The model under review builds one solid part; all positions refer to its coordinate system, in mm. Face numbers are marked on the shaded views. A direction names the side the tool comes from. Round coordinates to 2 decimals unless told otherwise and drop trailing zeros. Order: outer loops, then holes, each group sorted by start corner. A loop starts at its lowest first (then second) coordinate and runs counter-clockwise, first axis right, second up.
1) Clearance check with flat-ended pins moving along their axes: P1, Ø3.5, axis at x = -5, z = 7.5, coming from the +Y side; P2, Ø1, axis at y = 13, z = 14.5, coming from the -X side; P3, Ø1.1, axis at y = -2, z = 8.5, coming from the -X side. State where each tip first meets the part, or that it passes through.
2) To check wall thickness, follow L1, parallel to X at y = 45.5, z = 9.5; L2, parallel to Y at x = -120, z = 19.25; L3, parallel to Y at x = -16, z = 10.25. State the ranges of each line that lie inside material, in increasing order.
3) Mouldability with a two-part tool opening along Y and no side actions: class the marked faces 1, 2, 3 and 4 as pulls with the +Y half, pulls with the -Y half, needs draft (parallel to the pull), parting line crosses it, or undercut.
4) Machinability: for the marked faces 5, 6, 7, 8 and 9, which of the approach directions +Z, -Z, +X, -X, +Y, -Y give a long, thin tool a straight path to every point of the face, cutting with its end or side? Answer none if there is none.
5) Consider section C-C (x = -35). Give the boundary of the cut face in (y, z).
6) Consider section B-B (y = 43.5). Give the boundary of the cut face in (x, z).
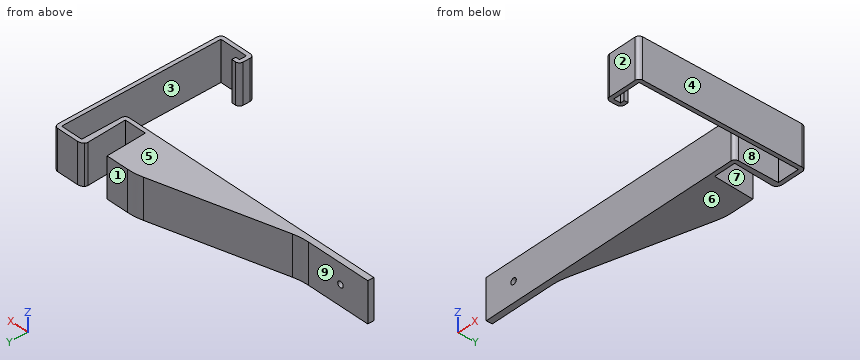
from build123d import *

# Parameters (mm, degrees)
F1_DEPTH = 20
F2_R     = 30
F3_R     = 2
F4_R     = 2
F5_R     = 1.5
F6_DEPTH = 25


with BuildPart() as f1:
    # F0 (on Top) → F1 (new body)
    with BuildSketch(Plane.XY):
        with BuildLine():
            Line((0, -3.5), (0, 0))
            Line((0, 0), (2, 0))
            Line((2, 0), (2, 2))
            Line((2, 2), (-2, 2))
            Line((-2, 2), (-2, 0))
            Line((-2, 0), (-2, -5.5))
            Line((-2, -5.5), (16, -5.5))
            Line((16, -5.5), (16, 54.5))
            Line((16, 54.5), (16, 76.5))
            ThreePointArc((16, 76.5), (15.414214, 77.914214), (14, 78.5))
            Line((14, 78.5), (3, 78.5))
            ThreePointArc((3, 78.5), (1.197224, 77.954163), (0, 76.5))
            Line((0, 76.5), (0.909091, 56.5))
            Line((0.909091, 56.5), (-10.090909, 56.5))
            Line((-10.090909, 56.5), (-11, 76.5))
            Line((-11, 76.5), (-26, 76.5))
            Line((-26, 76.5), (-96.908965, 57.5))
            Line((-96.908965, 57.5), (-133.387446, 57.5))
            Line((-133.387446, 57.5), (-133.387446, 54.5))
            Line((-133.387446, 54.5), (-10, 54.5))
            Line((-10, 54.5), (1, 54.5))
            Line((1, 54.5), (3, 54.5))
            Line((3, 54.5), (3, 76.5))
            Line((3, 76.5), (14, 76.5))
            Line((14, 76.5), (14, 54.5))
            Line((14, 54.5), (14, -3.5))
            Line((14, -3.5), (0, -3.5))
        make_face()
    extrude(amount=F1_DEPTH)

    # F2
    f2_edges = [f1.edges().sort_by_distance(p)[0] for p in [
        (-96.908965, 57.5, 10),
        (-26, 76.5, 10),
    ]]
    fillet(f2_edges, radius=F2_R)

    # F3
    f3_edges = [f1.edges().sort_by_distance(p)[0] for p in [
        (0, 76.5, 10),
    ]]
    fillet(f3_edges, radius=F3_R)

    # F4
    f4_edges = [f1.edges().sort_by_distance(p)[0] for p in [
        (16, -5.5, 10),
        (-2, -5.5, 10),
        (-2, 2, 10),
        (3, 54.5, 10),
    ]]
    fillet(f4_edges, radius=F4_R)

    # F5 (on face) → F6 (cut)
    with BuildSketch(Plane(origin=(0, 57.5, 0), x_dir=(-1, 0, 0), z_dir=(0, 1, 0))):
        with Locations((118.387446, 10)):
            Circle(F5_R)
    extrude(amount=-F6_DEPTH, mode=Mode.SUBTRACT)


solid = f1.part
Answer below:
1. P1: stops at y = 56.5
1. P2: stops at x = 14
1. P3: stops at x = -2
2. L1: x = 14 to 16
2. L2: y = 54.5 to 57.5
2. L3: y = 54.5 to 76.5
3. face 1: pulls with the +Y half
3. face 2: pulls with the -Y half
3. face 3: undercut
3. face 4: needs draft
4. face 5: +Z, +X, -X, +Y, -Y
4. face 6: -Z, +X, -X, +Y, -Y
4. face 7: +Z, -Z, +Y
4. face 8: +Z, -Z
4. face 9: +Z, -Z, -X, +Y
5. outline: (54.5, 0) - (74.09, 0) - (74.09, 20) - (54.5, 20) - close
6. outline: (14, 0) - (16, 0) - (16, 20) - (14, 20) - close
